from build123d import *

# Parameters (mm, degrees)
SKETCH4_R           = 7.5
BOSS_EXTRUDE1_DEPTH = 421
SKETCH5_R           = 6
BOSS_EXTRUDE2_DEPTH = 10
CHAMFER1_SIZE       = 0.5
SKETCH6_R           = 5
BOSS_EXTRUDE3_DEPTH = 30
SKETCH7_R           = 4
BOSS_EXTRUDE4_DEPTH = 15
CHAMFER2_SIZE       = 0.5


with BuildPart() as part:
    # Sketch4 → Boss-Extrude1 (new body)
    with BuildSketch(Plane(origin=(0, 0, 0), x_dir=(1, 0, 0), z_dir=(0, 1, 0))):
        Circle(SKETCH4_R)
    extrude(amount=BOSS_EXTRUDE1_DEPTH)

    # Sketch5 → Boss-Extrude2 (add)
    with BuildSketch(Plane(origin=(0, 421, 0), x_dir=(1, 0, 0), z_dir=(0, 1, 0))):
        Circle(SKETCH5_R)
    extrude(amount=BOSS_EXTRUDE2_DEPTH)

    # Chamfer1
    chamfer1_edges = [part.edges().sort_by_distance(p)[0] for p in [
        (-6, 431, 0),
    ]]
    chamfer(chamfer1_edges, length=CHAMFER1_SIZE)

    # Sketch6 → Boss-Extrude3 (add)
    with BuildSketch(Plane.XZ):
        Circle(SKETCH6_R)
    extrude(amount=BOSS_EXTRUDE3_DEPTH)

    # Sketch7 → Boss-Extrude4 (add)
    with BuildSketch(Plane.XZ.offset(30)):
        Circle(SKETCH7_R)
    extrude(amount=BOSS_EXTRUDE4_DEPTH)

    # Chamfer2
    chamfer2_edges = [part.edges().sort_by_distance(p)[0] for p in [
        (-4, -45, 0),
    ]]
    chamfer(chamfer2_edges, length=CHAMFER2_SIZE)


solid = part.part
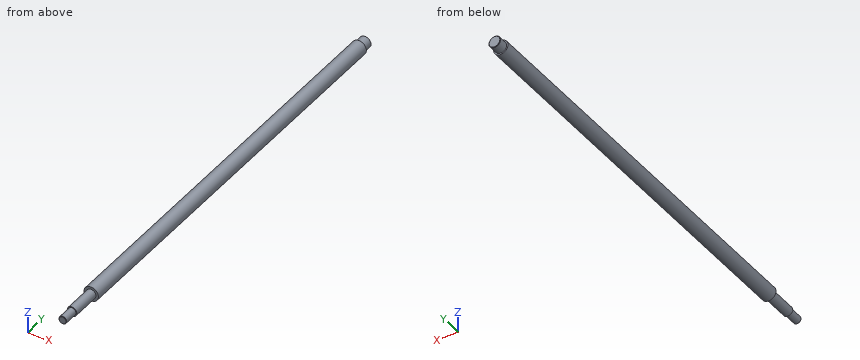
Input: part model. Units: mm. Frame: model coordinates. Give positions to 0.01 mm unless a question says otherwise; leave off trailing zeros. Order: outer loops, then holes, each group sorted by start corner. A loop starts at its lowest first (then second) coordinate and runs counter-clockwise, first axis right, second up. Notation, with made-up numbers: (58, -13.5) -> (100, -13.5) arc R16 cw to (100, -9.5) -> close; hole circle Ø5 at (79, -35.5). An arc over 180 degrees is marked (long way). Use one line per item in the form item = value.
1) Section B-B, the plane x = 0. Return loops of the section in (y, z), and give its area (3 significant figures).
Response values:
outline = (-45, -3.5) -> (-44.5, -4) -> (-30, -4) -> (-30, -5) -> (0, -5) -> (0, -7.5) -> (421, -7.5) -> (421, -6) -> (430.5, -6) -> (431, -5.5) -> (431, 5.5) -> (430.5, 6) -> (421, 6) -> (421, 7.5) -> (0, 7.5) -> (0, 5) -> (-30, 5) -> (-30, 4) -> (-44.5, 4) -> (-45, 3.5) -> close
area = 6,850 mm^2
2) Line query: probe 1 along X at (y, z) = (227, 5); probe 2 along Y at (x, z) = (-4, -3.75); probe 3 along Z at (x, y) = (0.5, 98). Output: solid intervals per line, ascending.
Response values:
probe_1 = -5.59 to 5.59
probe_2 = 0 to 431
probe_3 = -7.48 to 7.48
3) Section C-C, the plane y = 194. Return loops of the section in (x, z), and give its area (3 significant figures).
Response values:
outline = circle Ø15 at (0, 0)
area = 177 mm^2
4) First-contact query: pin 1 Ø6 at (x, y) = (-5, 272.5) entering from -Z; pin 2 Ø7.5 at (x, z) = (3.5, -2.5) entering from -Y; pin 3 Ø1.5 at (x, y) = (3.5, 67) entering from -Z; pin 4 Ø5 at (y, z) = (44.5, -5.5) entering from -X. Flat tips, straight axial feed; report the tip coordinate or a pass-through.
Response values:
pin_1 = -7.23
pin_2 = -45
pin_3 = -6.98
pin_4 = -6.87
5) Section A-A, the plane z = 0. Return loops of the section in (x, y).
Response values:
outline = (-7.5, 0) -> (-5, 0) -> (-5, -30) -> (-4, -30) -> (-4, -44.5) -> (-3.5, -45) -> (3.5, -45) -> (4, -44.5) -> (4, -30) -> (5, -30) -> (5, 0) -> (7.5, 0) -> (7.5, 421) -> (6, 421) -> (6, 430.5) -> (5.5, 431) -> (-5.5, 431) -> (-6, 430.5) -> (-6, 421) -> (-7.5, 421) -> close
